Input: part model. Units: mm. Frame: model coordinates. A direction names the side the tool comes from. Give positions to 0.01 mm unless a question says otherwise; leave off trailing zeros. Loops run counter-clockwise (first coordinate to the right, second up) from the corner with the lowest first, then second, coordinate; pieces in that order, holes last. Notation, with made-up numbers: (75.25, 11.25) -> (103.25, 11.25) arc R20 ccw to (103.25, 18.25) -> close; hole circle Ø11 at (40, 33.25). An arc over 180 degrees is marked (long way). Answer as a JSON object with one key per item and string values. Group by question number.
```python
from build123d import *

# Parameters (mm, degrees)
SKIZZE1_W                       = 125
SKIZZE1_H                       = 85
AUFSATZ_LINEAR_AUSTRAGEN1_DEPTH = 10
SKIZZE2_W                       = 100
SKIZZE2_H                       = 80
SCHNITT_LINEAR_AUSTRAGEN1_DEPTH = 5
SKIZZE3_W                       = 50
SKIZZE3_H                       = 50
AUFSATZ_LINEAR_AUSTRAGEN2_DEPTH = 2.5
SKIZZE4_R                       = 5
SCHNITT_LINEAR_AUSTRAGEN2_DEPTH = 22.5


with BuildPart() as part:
    # Skizze1 → Aufsatz-Linear austragen1 (new body)
    with BuildSketch(Plane.XY):
        with Locations((16.213851874, -21.700636943)):
            Rectangle(SKIZZE1_W, SKIZZE1_H)
    extrude(amount=AUFSATZ_LINEAR_AUSTRAGEN1_DEPTH)

    # Skizze2 → Schnitt-Linear austragen1 (cut)
    with BuildSketch(Plane.XY.offset(10)):
        with Locations((3.713851874, -24.200636943)):
            Rectangle(SKIZZE2_W, SKIZZE2_H)
    extrude(amount=-SCHNITT_LINEAR_AUSTRAGEN1_DEPTH, mode=Mode.SUBTRACT)

    # Skizze3 → Aufsatz-Linear austragen2 (add)
    with BuildSketch(Plane.XY.offset(5)):
        with Locations((-21.286148126, -24.200636943)):
            Rectangle(SKIZZE3_W, SKIZZE3_H)
    extrude(amount=AUFSATZ_LINEAR_AUSTRAGEN2_DEPTH)

    # Skizze4 → Schnitt-Linear austragen2 (cut)
    with BuildSketch(Plane.XY.offset(7.5)):
        with Locations((-36.286148126, -24.200636943)):
            Circle(SKIZZE4_R)
        with Locations((-16.286148126, -24.200636943)):
            Circle(SKIZZE4_R)
    extrude(amount=-SCHNITT_LINEAR_AUSTRAGEN2_DEPTH, mode=Mode.SUBTRACT)


solid = part.part
```
Q1. Pull-direction query (X, two-part tool) for faces 4 (the face through (-46.286, -22, 4)), 5 (the face through (15, 20.799, 5)), 6 (the face through (78.714, -22, 5)), 7 (the face through (53.714, -25, 8)); classes: +X half, -X half, draft (parallel to the pull), parting line (faces both ways), or undercut.
Q2. Section C-C on x = 44. Return the cut outline in (y, z).
Q3. Set-up query: faces 1 (the face through (-22, -24, 7.5)), 2 (the face through (3.714, -25, 6)), 3 (the face through (-22, 0.799, 6)). Return all of +Z, -Z, +X, -X, +Y, -Y with unobstructed straight access to the full face (end or side cutting, diameter ignored); none if empty.
Q4. Ray query, probe 1 along X at (y, z) = (-14, 6); probe 2 along Z at (x, y) = (-13, 5); probe 3 along Y at (x, z) = (-40, 1.25). Return the intervals inside material, ascending.
Q5. Section B-B on y = -16.5. Return the cut outline in (x, z).
Q6. Section D-D on y = 7.5. Return the cut outline in (x, z), then the cut area to 3 significant figures.
Q7. Section A-A on x = -15.5. Return the cut outline in (y, z), then the cut area to 3 significant figures.
Q8. Pin query (flat end, axial travel): pin 1 Ø8 at (x, y) = (-36.29, -24.2) entering from -Z; pin 2 Ø5 at (x, y) = (-11, -53.5) entering from +Z; pin 3 Ø2 at (x, z) = (1.5, 9) entering from -Y. Return the tip coordinate at first contact, or that it passes through.
Numbers:
{
 "1": {"face 4": "-X half", "face 5": "draft", "face 6": "+X half", "face 7": "undercut"},
 "2": {"outline": "(-64.2, 0) -> (20.8, 0) -> (20.8, 10) -> (15.8, 10) -> (15.8, 5) -> (-64.2, 5) -> close"},
 "3": {"face 1": "+Z, -X, -Y", "face 2": "+Z, -Y", "face 3": "+Z, -X"},
 "4": {"probe 1": "x = -46.29 to 3.71, 53.71 to 78.71", "probe 2": "z = 0 to 5", "probe 3": "y = -64.2 to -27.55, -20.85 to 20.8"},
 "5": {"outline": "(-46.29, 0) -> (78.71, 0) -> (78.71, 10) -> (53.71, 10) -> (53.71, 5) -> (3.71, 5) -> (3.71, 7.5) -> (-46.29, 7.5) -> close"},
 "6": {"outline": "(-46.29, 0) -> (78.71, 0) -> (78.71, 10) -> (53.71, 10) -> (53.71, 5) -> (-46.29, 5) -> close", "area": "750 mm²"},
 "7": {"outline": "(-64.2, 0) -> (-29.14, 0) -> (-29.14, 7.5) -> (-49.2, 7.5) -> (-49.2, 5) -> (-64.2, 5) -> close; (-19.26, 0) -> (20.8, 0) -> (20.8, 10) -> (15.8, 10) -> (15.8, 5) -> (0.8, 5) -> (0.8, 7.5) -> (-19.26, 7.5) -> close", "area": "501 mm²"},
 "8": {"pin 1": "passes through", "pin 2": "stops at z = 5", "pin 3": "stops at y = 15.8"}
}
